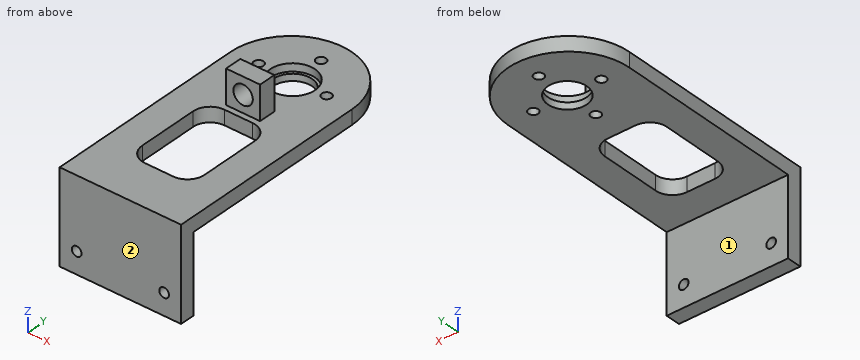
```python
from build123d import *

# Parameters (mm, degrees)
SKETCH1_W           = 25
SKETCH1_H           = 38.558203604
SKETCH1_H_2         = 3.441796396
BOSS_EXTRUDE1_DEPTH = 3
SKETCH2_R           = 4
SKETCH2_R_2         = 1
CUT_EXTRUDE1_DEPTH  = 3
SKETCH4_R           = 4.6
CUT_EXTRUDE2_DEPTH  = 1.6
SKETCH5_W           = 25
SKETCH5_H           = 3
BOSS_EXTRUDE3_DEPTH = 19
SKETCH7_R           = 1
CUT_EXTRUDE4_DEPTH  = 4
SKETCH8_W           = 12.783853214
SKETCH8_H           = 19.5
CUT_EXTRUDE5_DEPTH  = 4
FILLET1_R           = 3.5
SKETCH9_W           = 7
SKETCH9_H           = 3.5
BOSS_EXTRUDE4_DEPTH = 7
SKETCH10_R          = 2
CUT_EXTRUDE6_DEPTH  = 7


with BuildPart() as part:
    # Sketch1 → Boss-Extrude1 (new body)
    with BuildSketch(Plane.XY):
        with Locations((0, 8.156339421)):
            Rectangle(SKETCH1_W, SKETCH1_H)
        with BuildLine():
            Line((-12.5, 27.435441223), (12.5, 27.435441223))
            ThreePointArc((12.5, 27.435441223), (0, 39.935441223), (-12.5, 27.435441223))
        make_face()
        with Locations((0, -12.843660579)):
            Rectangle(SKETCH1_W, SKETCH1_H_2)
    extrude(amount=BOSS_EXTRUDE1_DEPTH)

    # Sketch2 → Cut-Extrude1 (cut)
    with BuildSketch(Plane.XY.offset(3)):
        with Locations((0, 27.802049159)):
            Circle(SKETCH2_R)
        with Locations((0, 34.802049159)):
            Circle(SKETCH2_R_2)
        with Locations((7, 27.802049159)):
            Circle(SKETCH2_R_2)
        with Locations((0, 20.802049159)):
            Circle(SKETCH2_R_2)
        with Locations((-7, 27.802049159)):
            Circle(SKETCH2_R_2)
    extrude(amount=-CUT_EXTRUDE1_DEPTH, mode=Mode.SUBTRACT)

    # Sketch4 → Cut-Extrude2 (cut)
    with BuildSketch(Plane.XY.offset(3)):
        with Locations((0, 27.802049159)):
            Circle(SKETCH4_R)
    extrude(amount=-CUT_EXTRUDE2_DEPTH, mode=Mode.SUBTRACT)

    # Sketch5 → Boss-Extrude3 (add)
    with BuildSketch(Plane.XY.offset(3)):
        with Locations((0, -13.064558777)):
            Rectangle(SKETCH5_W, SKETCH5_H)
    extrude(amount=-BOSS_EXTRUDE3_DEPTH)

    # Sketch7 → Cut-Extrude4 (cut)
    with BuildSketch(Plane(origin=(0, -11.564558777, 0), x_dir=(1, 0, 0), z_dir=(0, 1, 0))):
        with Locations((9, 11.55)):
            Circle(SKETCH7_R)
        with Locations((-9, 11.55)):
            Circle(SKETCH7_R)
    extrude(amount=-CUT_EXTRUDE4_DEPTH, mode=Mode.SUBTRACT)

    # Sketch8 → Cut-Extrude5 (cut)
    with BuildSketch(Plane.XY.offset(3)):
        with Locations((0, 4.716978639)):
            Rectangle(SKETCH8_W, SKETCH8_H)
    extrude(amount=-CUT_EXTRUDE5_DEPTH, mode=Mode.SUBTRACT)

    # Fillet1
    fillet1_edges = [part.edges().sort_by_distance(p)[0] for p in [
        (6.391926607, 14.466978639, 1.5),
        (6.391926607, -5.033021361, 1.5),
        (-6.391926607, -5.033021361, 1.5),
        (-6.391926607, 14.466978639, 1.5),
    ]]
    fillet(fillet1_edges, radius=FILLET1_R)

    # Sketch9 → Boss-Extrude4 (add)
    with BuildSketch(Plane.XY.offset(3)):
        with Locations((0, 17.365441223)):
            Rectangle(SKETCH9_W, SKETCH9_H)
    extrude(amount=BOSS_EXTRUDE4_DEPTH)

    # Sketch10 → Cut-Extrude6 (cut)
    with BuildSketch(Plane(origin=(0, 19.115441223, 0), x_dir=(1, 0, 0), z_dir=(0, 1, 0))):
        with Locations((0, -6.5)):
            Circle(SKETCH10_R)
    extrude(amount=-CUT_EXTRUDE6_DEPTH, mode=Mode.SUBTRACT)


solid = part.part
```
Source: CAD feature listing. Evaluate the final solid. Frame: model axes, mm. Face numbers are marked on the shaded views. A direction names the side the tool comes from. Give positions to 0.01 mm unless a question says otherwise; leave off trailing zeros. Loops run counter-clockwise (first coordinate to the right, second up) from the corner with the lowest first, then second, coordinate; pieces in that order, holes last. Notation, with made-up numbers: (58.25, 2) - (113.25, 2) arc R7 ccw to (113.25, 8) - close; hole circle Ø7 at (43.5, 74.5). An arc over 180 degrees is marked (long way). Use CSV: the item, a comma, the result in double quotes.
1) Line query: line 1 (Y direction, x = 0, z = 1.55); line 2 (Z direction, x = -9, y = -13.85); line 3 (Z direction, x = -8.75, y = 8.5). Output: solid intervals per line, ascending.
Worked out:
line 1,"y = -14.56 to -5.03, 14.47 to 19.8, 21.8 to 23.2, 32.4 to 33.8, 35.8 to 39.94"
line 2,"z = -16 to -12.55, -10.55 to 3"
line 3,"z = 0 to 3"
2) Pin query (flat end, axial travel): P1, Ø5, axis at x = 5.5, y = 2.5, coming from the -Z side; P2, Ø8, axis at x = -9, z = 4.5, coming from the +Y side; P3, Ø3, axis at x = 1, y = 28, coming from the +Z side; P4, Ø2.5, axis at x = 0, y = 20.8, coming from the +Z side. Return the tip coordinate at first contact, or that it passes through.
Worked out:
P1,"stops at z = 0"
P2,"stops at y = 38.76"
P3,"passes through"
P4,"stops at z = 3"
3) Cut plane B-B (x = 0). Count the separate pieces of the cut face and the enclosed holes in it, and give its area (3 significant figures).
Worked out:
separate pieces,"6"
enclosed holes,"0"
area,"126 mm^2"
4) Cut plane C-C (y = 16.5). Output: boundary loops of the cut face in (x, z), and give its area (3 significant figures).
Worked out:
outline,"(-12.5, 0) - (12.5, 0) - (12.5, 3) - (3.5, 3) - (3.5, 10) - (-3.5, 10) - (-3.5, 3) - (-12.5, 3) - close; hole circle Ø4 at (0, 6.5)"
area,"111 mm^2"
5) Cut plane D-D (x = -9). Output: boundary loops of the cut face in (y, z).
Worked out:
outline,"(-14.56, -16) - (-11.56, -16) - (-11.56, -12.55) - (-14.56, -12.55) - close; (-14.56, -10.55) - (-11.56, -10.55) - (-11.56, 0) - (36.11, 0) - (36.11, 3) - (-14.56, 3) - close"
6) Cut plane A-A (z = 6.5). Output: boundary loops of the cut face in (x, y).
Worked out:
outline,"(-3.5, 15.62) - (-2, 15.62) - (-2, 19.12) - (-3.5, 19.12) - close; (2, 15.62) - (3.5, 15.62) - (3.5, 19.12) - (2, 19.12) - close"
7) Set-up query: the marked faces 1 and 2. Return all of +Z, -Z, +X, -X, +Y, -Y with unobstructed straight access to the full face (end or side cutting, diameter ignored); none if empty.
Worked out:
face 1,"-Z, +X, -X, +Y"
face 2,"+Z, -Z, +X, -X, -Y"
